Geometry: final body of the model. Coordinates: model frame, mm. A direction names the side the tool comes from. Round coordinates to 2 decimals unless told otherwise and drop trailing zeros. Loops run counter-clockwise (first coordinate to the right, second up) from the corner with the lowest first, then second, coordinate; pieces in that order, holes last. Notation, with made-up numbers: (-33.75, 28) - (14.25, 28) arc R26 ccw to (14.25, 65) - close; hole circle Ø1 at (-31, 68). An arc over 180 degrees is marked (long way). Answer as CSV lines item,"result".
from build123d import *

# Parameters (mm, degrees)
F1_DEPTH = 12.7
F2_SIZE  = 2.54


with BuildPart() as f1:
    # F0 (on Front) → F1 (new body)
    with BuildSketch(Plane.XZ):
        Polygon((-24.902997, -61.232347), (0.497003, -61.232347), (0.497003, 40.367653), (38.597003, 40.367653), (38.597003, 27.667653), (51.297003, 27.667653), (51.297003, 72.117653), (-75.702997, 72.117653), (-75.702997, 27.667653), (-63.002997, 27.667653), (-63.002997, 40.367653), (-24.902997, 40.367653), align=None)
    extrude(amount=-F1_DEPTH)

    # F2
    f2_edges = [f1.edges().sort_by_distance(p)[0] for p in [
        (-12.202997, 0, 72.117653),
        (51.297003, 6.35, 72.117653),
        (-12.202997, 12.7, 72.117653),
        (-75.702997, 6.35, 72.117653),
        (51.297003, 6.35, 27.667653),
        (51.297003, 0, 49.892653),
        (51.297003, 12.7, 49.892653),
        (-75.702997, 6.35, 27.667653),
        (-75.702997, 0, 49.892653),
        (-75.702997, 12.7, 49.892653),
    ]]
    chamfer(f2_edges, length=F2_SIZE)


solid = f1.part
(1) Section A-A (y = 6). Output: boundary loops of the cut face in (x, z).
Findings below:
outline,"(-75.7, 30.21) - (-73.16, 27.67) - (-63, 27.67) - (-63, 40.37) - (-24.9, 40.37) - (-24.9, -61.23) - (0.5, -61.23) - (0.5, 40.37) - (38.6, 40.37) - (38.6, 27.67) - (48.76, 27.67) - (51.3, 30.21) - (51.3, 69.58) - (48.76, 72.12) - (-73.16, 72.12) - (-75.7, 69.58) - close"
(2) Section B-B (x = 11). Output: boundary loops of the cut face in (y, z).
Findings below:
outline,"(0, 40.37) - (12.7, 40.37) - (12.7, 69.58) - (10.16, 72.12) - (2.54, 72.12) - (0, 69.58) - close"
(3) Access query for faces 5 (the face through (-12, 6, -61.232)), 6 (the face through (44, 6, 27.668)), 7 (the face through (-68, 6, 27.668)), 8 (the face through (38.597, 6, 34)), 9 (the face through (-13, 12.7, 34)). Directions: +Z, -Z, +X, -X, +Y, -Y. A direction counts if a zero-diameter tool reaches every point of the face in a straight line with its end or side. Return the directions, or none.
Findings below:
face 5,"-Z, +X, -X, +Y, -Y"
face 6,"-Z, +X, +Y, -Y"
face 7,"-Z, -X, +Y, -Y"
face 8,"-Z, +Y, -Y"
face 9,"+Z, -Z, +X, -X, +Y"
(4) Draft query along X for faces 1 (the face through (-13, 0, 34)), 2 (the face through (-75.703, 6, 50)), 3 (the face through (-63.003, 6, 34)), 4 (the face through (51.297, 6, 50)). Return one class per face: pulls with the +X half, pulls with the -X half, needs draft (parallel to the pull), parting line crosses it, or undercut.
Findings below:
face 1,"needs draft"
face 2,"pulls with the -X half"
face 3,"undercut"
face 4,"pulls with the +X half"
(5) Pin query (flat end, axial travel): P1, Ø6.5, axis at y = 4, z = -10.5, coming from the -X side; P2, Ø5, axis at x = -68, y = 4, coming from the -Z side; P3, Ø1.5, axis at x = -27, y = 9, coming from the -Z side. Return the tip coordinate at first contact, or that it passes through.
Findings below:
P1,"x = -24.9"
P2,"z = 27.67"
P3,"z = 40.37"
(6) Material intervals for line 1 along X through (y, z) = (6.75, 31.5); line 2 along X through (y, z) = (5.5, 3.5); line 3 along Z through (x, y) = (-68.5, 9.25), sorted ascending.
Findings below:
line 1,"-75.7 to -63, -24.9 to 0.5, 38.6 to 51.3"
line 2,"-24.9 to 0.5"
line 3,"27.67 to 72.12"
(7) Section C-C (z = -20). Output: boundary loops of the cut face in (x, y).
Findings below:
outline,"(-24.9, 0) - (0.5, 0) - (0.5, 12.7) - (-24.9, 12.7) - close"
